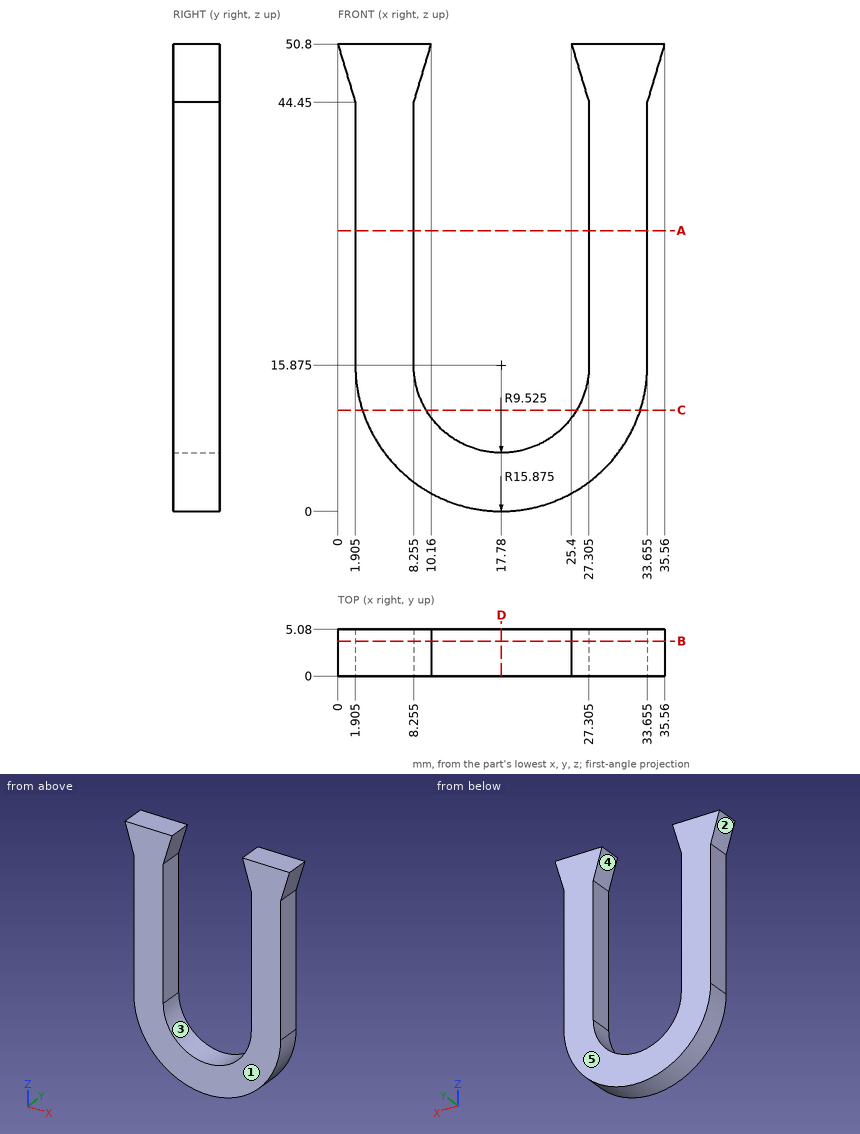
Design review of the part shown in the three views and the two pictorial views. Dimensions are in mm from the part's minimum x, y and z. A direction names the side the tool comes from. Round coordinates to 2 decimals unless told otherwise and drop trailing zeros. Loops run counter-clockwise (first coordinate to the right, second up) from the corner with the lowest first, then second, coordinate; pieces in that order, holes last.
(1) Clearance check with flat-ended pins moving along their axes: P1, Ø1.5, axis at x = 31, y = 0.5, coming from the -Z side; P2, Ø2.5, axis at y = 1.5, z = 29.5, coming from the -X side (3 decimals); P3, Ø1, axis at y = 2.5, z = 14, coming from the -X side. State where each tip first meets the part, or that it passes through.
Returned:
P1: stops at z = 6.05
P2: stops at x = 1.905
P3: stops at x = 1.96
(2) We need section D-D (x = 17.78). Give the boundary of the cut face in (y, z), plus the area to 3 significant figures.
Returned:
outline: (0, 0) - (5.08, 0) - (5.08, 6.35) - (0, 6.35) - close
area: 32.3 mm2
(3) Tool access review of the marked faces 4 and 5: name each direction out of +Z, -Z, +X, -X, +Y, -Y from which nothing blocks a thin tool from reaching the whole face with its end or side.
Returned:
face 4: +Y, -Y
face 5: +Z, -Z, +X, -X, +Y
(4) We need section C-C (z = 11). Give the boundary of the cut face in (x, y), plus the area to 3 significant figures.
Returned:
outline: (2.67, 0) - (9.6, 0) - (9.6, 5.08) - (2.67, 5.08) - close; (25.96, 0) - (32.89, 0) - (32.89, 5.08) - (25.96, 5.08) - close
area: 70.4 mm2
(5) Mouldability with a two-part tool opening along X and no side actions: class the marked faces 1, 2 and 3 as released by +X, released by -X, zero draft, split by the parting line, or undercut.
Returned:
face 1: zero draft
face 2: released by -X
face 3: undercut
(6) Wall thickness on line 1 along X through (y, z) = (0.4, 35) (3 decimals); line 2 along X through (y, z) = (4.65, 13); line 3 along Z through (x, y) = (15.5, 2.1): over which ranges is each line inside the solid? List them lowest first.
Returned:
line 1: x = 1.905 to 8.255, 27.305 to 33.655
line 2: x = 2.17 to 8.7, 26.86 to 33.39
line 3: z = 0.16 to 6.63
(7) We need section B-B (y = 3.8). Give the boundary of the cut face in (x, z) (3 decimals).
Returned:
outline: (0, 50.8) - (1.905, 44.45) - (1.905, 15.875) arc R15.875 ccw to (33.655, 15.875) - (33.655, 44.45) - (35.56, 50.8) - (25.4, 50.8) - (27.305, 44.45) - (27.305, 15.875) arc R9.525 cw to (8.255, 15.875) - (8.255, 44.45) - (10.16, 50.8) - close
(8) We need section A-A (z = 30.5). Give the boundary of the cut face in (x, y) (3 decimals), plus the area to 3 significant figures.
Returned:
outline: (1.905, 0) - (8.255, 0) - (8.255, 5.08) - (1.905, 5.08) - close; (27.305, 0) - (33.655, 0) - (33.655, 5.08) - (27.305, 5.08) - close
area: 64.5 mm2
